Drawing for the job (mm, zero at the part's lowest x, y, z). A direction names the side the tool comes from. Coordinates: 2 decimals unless noted, no trailing zeros. Order: outer loops, then holes, each group sorted by start corner. A loop starts at its lowest first (then second) coordinate and runs counter-clockwise, first axis right, second up. Notation, with made-up numbers: M 14,43 L 46,43 A8 cw 46,58 Z; hole C -11.75,72.5 d4. An arc over 180 degrees is marked long. Write item = value, one per line. Start each with the question number.
Q1. Band-saw the part on D-D on x = 19. Write the cut outline in (y, z), plus the area to 3 significant figures.
Q2. Pin check, flat tip, straight feed: P1, Ø7.5, axis at x = 21, y = 7.5, coming from the -Z side. Stop position of the tip, or through.
Q3. Band-saw the part on C-C on y = 13.25. Write the cut outline in (x, z), plus the area to 3 significant figures.
Q4. Band-saw the part on B-B on z = 19.7. Write the cut outline in (x, y), plus the area to 3 significant figures.
Q5. Band-saw the part on A-A on x = 25.5. Write the cut outline in (y, z), plus the area to 3 significant figures.
Q6. Drill centre lines: probe 1 along Y at (x, z) = (12.8, 32.05); probe 2 along Z at (x, y) = (0.25, 7.5); probe 3 along Z at (x, y) = (22.5, 14). Where is each one in solid material? Low to high.
Q7. 3-axis set-ups, long thin cutter, end or side, ignore diameter. For the marked faces 1 and 2: which of +Z, -Z, +X, -X, +Y, -Y reach the whole face in a straight line?
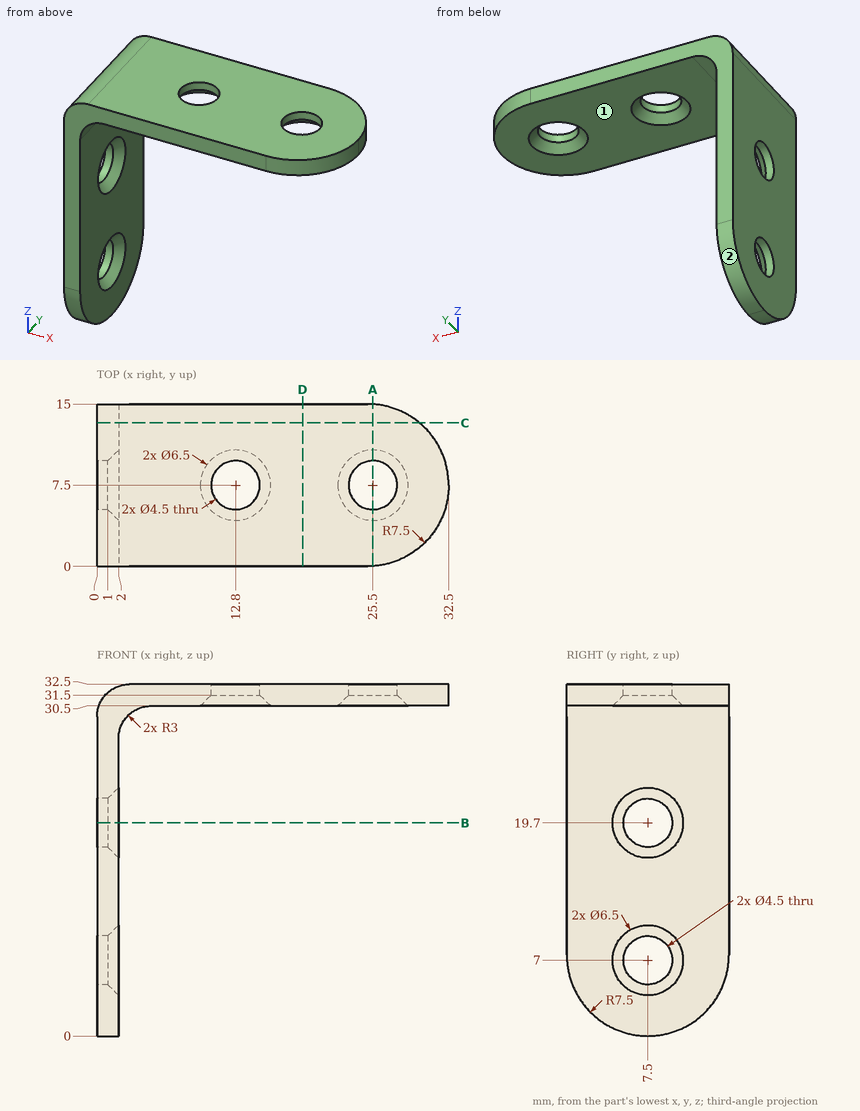
Recorded:
q1.outline = M 0,30.5 L 15,30.5 L 15,32.5 L 0,32.5 Z
q1.area = 30.0 mm2
q2.P1 = 30.5
q3.outline = M 0,2.68 L 2,2.68 L 2,27.5 A3 cw 5,30.5 L 29.82,30.5 L 29.82,32.5 L 3,32.5 A3 ccw 0,29.5 Z
q3.area = 115 mm2
q4.outline = M 0,0 L 2,0 L 2,4.25 L 1,5.25 L 0,5.25 Z; M 0,9.75 L 1,9.75 L 2,10.75 L 2,15 L 0,15 Z
q4.area = 20.0 mm2
q5.outline = M 0.02,30.5 L 4.25,30.5 L 5.25,31.5 L 5.25,32.5 L 0.02,32.5 Z; M 9.75,31.5 L 10.75,30.5 L 14.98,30.5 L 14.98,32.5 L 9.75,32.5 Z
q5.area = 19.9 mm2
q6.probe_1 = 0 to 5.25, 9.75 to 15
q6.probe_2 = 0 to 4.75, 9.25 to 17.45, 21.95 to 30.7
q6.probe_3 = 30.5 to 32.5
q7.face_1 = -Z, +X, +Y, -Y
q7.face_2 = -Z, +X, -X, +Y
